For this review, take the finished solid that the model builds, in its own axes (mm). Coordinates: 2 decimals unless noted, no trailing zeros. Loops run counter-clockwise (first coordinate to the right, second up) from the corner with the lowest first, then second, coordinate; pieces in that order, holes last.
Autodesk Inventor part; units mm, degrees
ref_plane "YZ Plane" through (0, 0, 0) normal (1, 0, 0) x (0, 1, 0)
ref_plane "XZ Plane" through (0, 0, 0) normal (0, 1, 0) x (-1, 0, 0)
ref_plane "XY Plane" through (0, 0, 0) normal (0, 0, 1) x (1, 0, 0)
sketch "Esquisse1" plane through (0, 0, 0) normal (0, 1, 0) x (-1, 0, 0)
  line L0 (0, 0) -> (10, 0)
  line L1 (10, 0) -> (10, -22)
  line L2 (10, -22) -> (0, -22)
  line L3 (0, -22) -> (0, 0)
  line L4 (5, 0) -> (5, -22) construction
  line L5 (10, -11) -> (0, -11) construction
  circle A0 centre (5, -11) radius 2.05
  circle A1 centre (5, -17) radius 2.05
  circle A2 centre (5, -5) radius 2.05
  dimension "d0" = 4.1
  dimension "d1" = 5
  dimension "d2" = 6
  dimension "d3" = 5
extrude "Extrusion1" add sketch "Esquisse1" along normal blind 3
fillet "Congé1" radius 2 4 edges at (-10, 1.5, 0) (0, 1.5, 0) (0, 1.5, -22) (-10, 1.5, -22)
equation "\"d3\" = d1"
properties part number "spacer"
Q1. Consider section B-B (x = -6.75). State the section outline as (y, z) points.
Q2. Consider section D-D (x = -5). State the section outline as (y, z) points, then the cut area to 3 significant figures.
Q3. Wall thickness on probe 1 along Z at (x, y) = (-5, 1.3); probe 2 along Z at (x, y) = (-6.5, 0.75); probe 3 along X at (y, z) = (1.2, -6.5): over which ranges is each line inside the solid? List them lowest first.
Q4. The part is to be moulded in two halves that separate along X. For faces 1 (the face through (-10, 1, -11)), 2 (the face through (-2.95, 1.48, -5.09)), 3 (the face through (0, 1, -11)), say which applies: +X half, -X half, draft (parallel to the pull), parting line (faces both ways), or undercut.
Q5. Consider section C-C (y = 0.5). State the section outline as (x, z) points.
Q6. Consider section A-A (z = -17). State the section outline as (x, y) points.
Model answer:
1. outline: (0, -22) - (3, -22) - (3, -18.07) - (0, -18.07) - close; (0, -15.93) - (3, -15.93) - (3, -12.07) - (0, -12.07) - close; (0, -9.93) - (3, -9.93) - (3, -6.07) - (0, -6.07) - close; (0, -3.93) - (3, -3.93) - (3, 0) - (0, 0) - close
2. outline: (0, -22) - (3, -22) - (3, -19.05) - (0, -19.05) - close; (0, -14.95) - (3, -14.95) - (3, -13.05) - (0, -13.05) - close; (0, -8.95) - (3, -8.95) - (3, -7.05) - (0, -7.05) - close; (0, -2.95) - (3, -2.95) - (3, 0) - (0, 0) - close
2. area: 29.1 mm2
3. probe 1: z = -22 to -19.05, -14.95 to -13.05, -8.95 to -7.05, -2.95 to 0
3. probe 2: z = -22 to -18.4, -15.6 to -12.4, -9.6 to -6.4, -3.6 to 0
3. probe 3: x = -10 to -6.4, -3.6 to 0
4. face 1: -X half
4. face 2: undercut
4. face 3: +X half
5. outline: (-10, -20) arc R2 ccw to (-8, -22) - (-2, -22) arc R2 ccw to (0, -20) - (0, -2) arc R2 ccw to (-2, 0) - (-8, 0) arc R2 ccw to (-10, -2) - close; hole circle Ø4.1 at (-5, -17); hole circle Ø4.1 at (-5, -11); hole circle Ø4.1 at (-5, -5)
6. outline: (-10, 0) - (-7.05, 0) - (-7.05, 3) - (-10, 3) - close; (-2.95, 0) - (0, 0) - (0, 3) - (-2.95, 3) - close
